from build123d import *

# Parameters (mm, degrees)
F0_R     = 28.575
F0_R_2   = 25.4
F0_R_3   = 31.75
F3_DEPTH = 3.175


# Not quite as in the source:
# - a fillet or chamfer that OpenCascade refuses, or shapes differently, is made with other operations: its cross-section is extruded or revolved along the edge and cut away or added


with BuildPart() as f2:
    # F2: sweep along a path in F1
    with BuildLine(Plane.YZ) as f2_path:
        Line((0, 0), (101.6, 0))
    # F0 (on Front) → F2 (sweep)
    with BuildSketch(Plane.XZ):
        Circle(F0_R)
        Circle(F0_R_2, mode=Mode.SUBTRACT)
    sweep(path=f2_path.line)

    # F0 (on Front) → F3 (join)
    with BuildSketch(Plane.XZ):
        Circle(F0_R_3)
        Circle(F0_R, mode=Mode.SUBTRACT)
    extrude(amount=-F3_DEPTH)

    # F1 (on Right) → F4 (revolve)
    with BuildSketch(Plane.YZ):
        Polygon((96.52, 28.575), (101.6, 28.575), (121.92, 28.575), (121.92, 31.75), (96.52, 31.75), align=None)
    revolve(axis=Axis((0, 50.8, 0), (0, 1, 0)))

    # F5: fillet of radius 5.08 on 2 edges, made by hand

    # F5_s1 → F5_t2 (revolve, cut)
    with BuildSketch(Plane.XY):
        with BuildLine():
            ThreePointArc((28.575, 101.6), (26.2678865162, 99.7305202921), (25.4, 96.8907139607))
            Line((25.4, 96.8907139607), (25.4, 101.6))
            Line((25.4, 101.6), (28.575, 101.6))
        make_face()
    revolve(axis=Axis((0, 101.6, 0), (0, 1, 0)), mode=Mode.SUBTRACT)

    # F5_s3 → F5_t4 (revolve, cut)
    with BuildSketch(Plane.YZ):
        with BuildLine():
            ThreePointArc((96.52, 28.575), (98.3894797079, 30.8821134838), (101.2292860393, 31.75))
            Line((101.2292860393, 31.75), (96.52, 31.75))
            Line((96.52, 31.75), (96.52, 28.575))
        make_face()
    revolve(axis=Axis((0, 96.52, 0), (0, 1, 0)), mode=Mode.SUBTRACT)


solid = f2.part
Read the model definition and answer for the solid it produces. Units are mm, in the model's axes. A direction names the side the tool comes from. Round coordinates to 2 decimals unless told otherwise and drop trailing zeros. Order: outer loops, then holes, each group sorted by start corner. A loop starts at its lowest first (then second) coordinate and runs counter-clockwise, first axis right, second up.
1) Straight lines are drawn through the part: L1, parallel to X at y = 117.25, z = 0 (3 decimals); L2, parallel to X at y = 36.5, z = 0 (3 decimals). For each, find the intervals that lie inside material, in ascending order.
2) For faces 1 (the face through (8.583, 111.902, 27.255)), 2 (the face through (-30.995, 111.43, -6.883)), 3 (the face through (-28.4, 3.175, 4.9)), determine the directions among +Z, -Z, +X, -X, +Y, -Y from which every point of the face is accessible in a straight line to the end or side of a thin tool.
3) The part is cut by section A-A on z = 0. Write down the section's boundary in (x, y) (3 decimals).
4) The part is cut by section C-C on y = 68. Write down the section's boundary in (x, z) (3 decimals), plus the area to 3 significant figures.
5) Flat-ended cylindrical pins translate along their axes: pin 1 (1 mm diameter, centred on x = -7, y = 62.5, fed in from +Z); pin 2 (1.5 mm diameter, centred on x = -21, z = 14.5, fed in from +Y); pin 3 (2 mm diameter, centred on x = -21.5, y = 108.5, fed in from -Z). Find the tip coordinate at first contact, or state that the pin passes through.
6) The mould has two halves that part along Y. Classify faces 4 (the face through (4.9, 121.92, 28.4)), 5 (the face through (26.4, 50.5, 10.94)), 6 (the face through (-14.3, 0, 21.3)), 7 (the face through (-6.883, 1.565, -30.995)): released by +Y, released by -Y, zero draft, split by the parting line, or undercut.
7) The part is cut by section B-B on x = 0. Write down the section's boundary in (y, z) (3 decimals), plus the area to 3 significant figures.
Resolved:
1. L1: x = -31.75 to -28.575, 28.575 to 31.75
1. L2: x = -28.575 to -25.4, 25.4 to 28.575
2. face 1: +Y
2. face 2: +Y, -Y
2. face 3: none
3. outline: (-31.75, 0) - (-25.4, 0) - (-25.4, 96.891) arc R5.08 ccw to (-28.575, 101.6) - (-28.575, 121.92) - (-31.75, 121.92) - (-31.75, 101.229) arc R5.08 ccw to (-28.575, 96.52) - (-28.575, 3.175) - (-31.75, 3.175) - close; (25.4, 0) - (31.75, 0) - (31.75, 3.175) - (28.575, 3.175) - (28.575, 96.52) arc R5.08 ccw to (31.75, 101.229) - (31.75, 121.92) - (28.575, 121.92) - (28.575, 101.6) arc R5.08 ccw to (25.4, 96.891) - close
4. outline: circle Ø57.15 at (0, 0); hole circle Ø50.8 at (0, 0)
4. area: 538 mm2
5. pin 1: stops at z = 27.83
5. pin 2: stops at y = 99.73
5. pin 3: stops at z = -24.24
6. face 4: released by +Y
6. face 5: undercut
6. face 6: released by -Y
6. face 7: zero draft
7. outline: (0, -31.75) - (3.175, -31.75) - (3.175, -28.575) - (96.52, -28.575) arc R5.08 ccw to (101.229, -31.75) - (121.92, -31.75) - (121.92, -28.575) - (101.6, -28.575) arc R5.08 ccw to (96.891, -25.4) - (0, -25.4) - close; (0, 25.4) - (96.891, 25.4) arc R5.08 ccw to (101.6, 28.575) - (121.92, 28.575) - (121.92, 31.75) - (101.229, 31.75) arc R5.08 ccw to (96.52, 28.575) - (3.175, 28.575) - (3.175, 31.75) - (0, 31.75) - close
7. area: 810 mm2
